For this review, take the finished solid that the model builds, in its own axes (mm). Give positions to 0.01 mm unless a question says otherwise; leave off trailing zeros. Loops run counter-clockwise (first coordinate to the right, second up) from the corner with the lowest first, then second, coordinate; pieces in that order, holes last. Notation, with made-up numbers: (43, 29.5) - (79, 29.5) arc R18 ccw to (79, 44.5) - close; hole circle Ø3 at (-35, 24). An arc over 180 degrees is marked (long way). Use CSV: the item, a comma, the result in double quotes. Start each with the question number.
1. Take a section at A-A on y = 122.5. Give the boundary of the cut face in (x, z) (3 decimals).
2. Wall thickness on line 1 (X direction, y = 85.5, z = 17.5) (3 decimals): over which ranges is the line inside the solid? List them lowest first.
3. For pin 1 (9.5 mm diameter, centred on x = 8.5, z = 6.5, fed in from -Y) (3 decimals); pin 2 (9.5 mm diameter, centred on x = 13, z = 5.5, fed in from +Y) (3 decimals); pin 3 (8 mm diameter, centred on y = 86, z = 7.5, fed in from -X), all flat-tipped, find the tip position at first contact; note any pin that passes through.
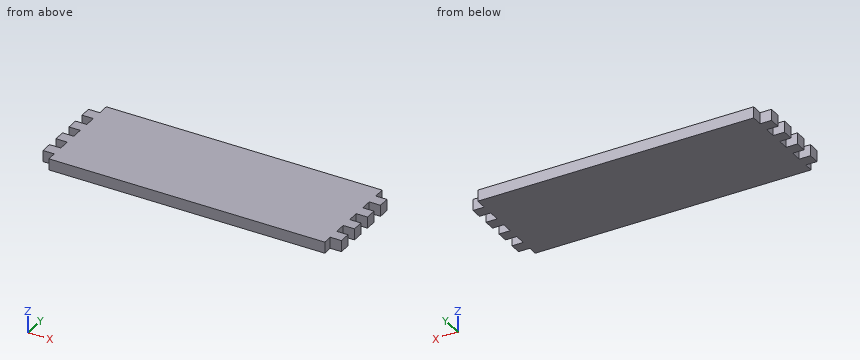
Autodesk Inventor part; units mm, degrees
ref_plane "YZ Plane" through (0, 0, 0) normal (1, 0, 0) x (0, 1, 0)
ref_plane "XZ Plane" through (0, 0, 0) normal (0, 1, 0) x (-1, 0, 0)
ref_plane "XY Plane" through (0, 0, 0) normal (0, 0, 1) x (1, 0, 0)
sketch "Sketch1" plane through (0, 0, 0) normal (0, 0, 1) x (1, 0, 0)
  line L0 (0, 0) -> (252.4125, 0)
  line L1 (252.4125, 0) -> (252.4125, 244.475)
  line L2 (252.4125, 244.475) -> (0, 244.475)
  line L3 (0, 244.475) -> (0, 0)
  dimension "d0" = 252.4125
  dimension "d1" = 244.475
extrude "Extrusion1" add sketch "Sketch1" along normal blind 19.05
sketch "Sketch3" plane through (0, 0, 19.05) normal (0, 0, 1) x (1, 0, 0)
  line L0 (0, 0) -> (252.4125, 0)
  line L1 (252.4125, 244.475) -> (0, 244.475)
  line L2 (0, 244.475) -> (0, 0)
  line L3 (0, 244.475) -> (19.05, 244.475)
  line L4 (19.05, 244.475) -> (19.05, 225.425)
  line L5 (19.05, 225.425) -> (0, 225.425)
  line L6 (0, 225.425) -> (0, 244.475)
  line L7 (19.05, 168.275) -> (0, 168.275)
  line L8 (0, 168.275) -> (0, 149.225)
  line L9 (0, 149.225) -> (19.05, 149.225)
  line L10 (19.05, 149.225) -> (19.05, 168.275)
  line L11 (0, 130.175) -> (19.05, 130.175)
  line L12 (19.05, 130.175) -> (19.05, 111.125)
  line L13 (19.05, 111.125) -> (0, 111.125)
  line L14 (0, 111.125) -> (0, 130.175)
  line L15 (0, 206.375) -> (19.05, 206.375)
  line L16 (19.05, 206.375) -> (19.05, 187.325)
  line L17 (19.05, 187.325) -> (0, 187.325)
  line L18 (0, 187.325) -> (0, 206.375)
  line L19 (0, 92.075) -> (19.05, 92.075)
  line L20 (19.05, 92.075) -> (19.05, 73.025)
  line L21 (19.05, 73.025) -> (0, 73.025)
  line L22 (0, 73.025) -> (0, 92.075)
  line L23 (0, 53.975) -> (19.05, 53.975)
  line L24 (19.05, 53.975) -> (19.05, 34.925)
  line L25 (19.05, 34.925) -> (0, 34.925)
  line L26 (0, 34.925) -> (0, 53.975)
  line L27 (0, 15.875) -> (19.05, 15.875)
  line L28 (19.05, 15.875) -> (19.05, -3.175)
  line L29 (19.05, -3.175) -> (0, -3.175)
  line L30 (0, -3.175) -> (0, 15.875)
  dimension "d4" = 19.05
  dimension "d5" = 19.05
  dimension "d6" = 244.475
  dimension "d7" = 19.05
  dimension "d8" = 19.05
  dimension "d9" = 19.05
  dimension "d10" = 19.05
  dimension "d11" = 19.05
  dimension "d12" = 19.05
  dimension "d13" = 19.05
  dimension "d14" = 19.05
  dimension "d15" = 19.05
  dimension "d16" = 19.05
  dimension "d17" = 19.05
  dimension "d18" = 19.05
  dimension "d19" = 19.05
  dimension "d20" = 19.05
  dimension "d21" = 19.05
  dimension "d22" = 19.05
  dimension "d23" = 19.05
  dimension "d24" = 15.875
extrude "Extrusion2" cut sketch "Sketch3" against normal through all
mirror "Mirror1" about plane through (252.4125, 0, 0) normal (1, 0, 0)
sketch "Sketch6" plane through (0, 0, 19.05) normal (0, 0, 1) x (1, 0, 0)
  line L0 (19.05, 34.925) -> (0, 34.925)
  line L1 (0, 34.925) -> (0, 15.875)
  line L2 (0, 15.875) -> (19.05, 15.875)
  line L3 (19.05, 15.875) -> (19.05, 0)
  line L4 (19.05, 0) -> (485.775, 0)
  line L5 (485.775, 15.875) -> (485.775, 0)
  line L6 (504.825, 15.875) -> (485.775, 15.875)
  line L7 (504.825, 34.925) -> (504.825, 15.875)
  line L8 (485.775, 34.925) -> (504.825, 34.925)
  line L9 (485.775, 53.975) -> (485.775, 34.925)
  line L10 (504.825, 53.975) -> (485.775, 53.975)
  line L11 (504.825, 73.025) -> (504.825, 53.975)
  line L12 (485.775, 73.025) -> (504.825, 73.025)
  line L13 (485.775, 92.075) -> (485.775, 73.025)
  line L14 (19.05, 92.075) -> (19.05, 73.025)
  line L15 (19.05, 73.025) -> (0, 73.025)
  line L16 (0, 73.025) -> (0, 53.975)
  line L17 (0, 53.975) -> (19.05, 53.975)
  line L18 (19.05, 53.975) -> (19.05, 34.925)
  line L19 (504.825, 76.2) -> (19.05, 76.2)
  line L20 (19.05, 76.2) -> (485.775, 76.2)
  line L21 (19.05, 244.475) -> (485.775, 244.475)
  point P0 (0, 0)
  dimension "d54" = 168.275
extrude "Extrusion3" cut sketch "Sketch6" against normal through all
properties part number "deep_side" material "Wood (Birch)"
Check result:
1,outline,"(19.05, 0) - (485.775, 0) - (485.775, 19.05) - (19.05, 19.05) - close"
2,line 1,"x = 19.05 to 485.775"
3,pin 1,"stops at y = 92.075"
3,pin 2,"stops at y = 225.425"
3,pin 3,"stops at x = 19.05"
